Source: CAD feature listing. Evaluate the final solid. Frame: model axes, mm. A direction names the side the tool comes from. Give positions to 0.01 mm unless a question says otherwise; leave off trailing zeros. Order: outer loops, then holes, each group sorted by start corner. A loop starts at its lowest first (then second) coordinate and runs counter-clockwise, first axis right, second up. Notation, with made-up numbers: M 67,-7.5 L 104,-7.5 A23 ccw 104,23.5 Z; hole C 70.25,28.5 d11. An arc over 180 degrees is marked long. Answer in a Markdown table with one row per item. Add a question column.
(1) Mould query, pull axis X, two halves, no side actions, for faces 3 (the face through (0, -1.025, 3)), 4 (the face through (0, 2, 6.25)), 5 (the face through (-7.5, 0, 3)), 6 (the face through (-2.65, 0, 3)). Classes: pulls with the +X half, pulls with the -X half, needs draft (parallel to the pull), parting line crosses it, or undercut.
(2) Section query C-C, the plane y = -0.2. Return loops of the section in (x, z) (3 decimals), plus the area to 3 significant figures.
(3) Section query A-A, the plane x = 5. Return loops of the section in (y, z) (3 decimals).
(4) Pin query (flat end, axial travel): P1, Ø1.4, axis at x = -5, z = 3.125, coming from the -Y side. Return the tip coordinate at first contact, or that it passes through.
(5) Material intervals for line 1 along Y through (x, z) = (1.5, 1.75) (3 decimals); line 2 along X through (y, z) = (0.35, 4.5); line 3 along Z through (x, y) = (-5, -0.7) (3 decimals), sorted ascending.
(6) Set-up query: faces 1 (the face through (7.5, 0, 3)), 2 (the face through (0, 1.025, 3)). Return all of +Z, -Z, +X, -X, +Y, -Y with unobstructed straight access to the full face (end or side cutting, diameter ignored); none if empty.
(7) Section query B-B, the plane z = 4.25. Return loops of the section in (x, y) (3 decimals), plus the area to 3 significant figures.
from build123d import *

# Parameters (mm, degrees)
F0_W     = 15
F0_H     = 5
F0_W_2   = 5.3
F0_H_2   = 2.05
F1_DEPTH = 6.25
F2_R     = 0.75
F3_DEPTH = 3.9


with BuildPart() as f1:
    # F0 (on Top) → F1 (new body)
    with BuildSketch(Plane.XY):
        Rectangle(F0_W, F0_H)
        Rectangle(F0_W_2, F0_H_2, mode=Mode.SUBTRACT)
    extrude(amount=F1_DEPTH)

    # F2 (on Front) → F3 (cut, symmetric)
    with BuildSketch(Plane.XZ):
        with Locations((-5, 3.125)):
            Circle(F2_R)
        with Locations((5, 3.125)):
            Circle(F2_R)
    extrude(amount=F3_DEPTH, both=True, mode=Mode.SUBTRACT)


solid = f1.part
Values follow:
| question | item | result |
|---|---|---|
| 1 | face 3 | undercut |
| 1 | face 4 | needs draft |
| 1 | face 5 | pulls with the -X half |
| 1 | face 6 | undercut |
| 2 | outline | M -7.5,0 L -2.65,0 L -2.65,6.25 L -7.5,6.25 Z; M 2.65,0 L 7.5,0 L 7.5,6.25 L 2.65,6.25 Z; hole C -5,3.125 d1.5; hole C 5,3.125 d1.5 |
| 2 | area | 57.1 mm² |
| 3 | outline | M -2.5,0 L 2.5,0 L 2.5,2.375 L -2.5,2.375 Z; M -2.5,3.875 L 2.5,3.875 L 2.5,6.25 L -2.5,6.25 Z |
| 4 | P1 | passes through |
| 5 | line 1 | y = -2.5 to -1.025, 1.025 to 2.5 |
| 5 | line 2 | x = -7.5 to -2.65, 2.65 to 7.5 |
| 5 | line 3 | z = 0 to 2.375, 3.875 to 6.25 |
| 6 | face 1 | +Z, -Z, +X, +Y, -Y |
| 6 | face 2 | +Z, -Z |
| 7 | outline | M -7.5,-2.5 L 7.5,-2.5 L 7.5,2.5 L -7.5,2.5 Z; hole M -2.65,-1.025 L 2.65,-1.025 L 2.65,1.025 L -2.65,1.025 Z |
| 7 | area | 64.1 mm² |
